```python
from build123d import *

# Parameters (mm, degrees)
BOSS_EXTRUDE1_DEPTH     = 20
BOSS_EXTRUDE2_START     = -5
BOSS_EXTRUDE2_DEPTH     = 5
CUT_EXTRUDE1_DEPTH      = 295.553899991
CUT_EXTRUDE1_DEPTH_BACK = 295.553899991
SKETCH3_R               = 1.5
SKETCH4_R               = 29
BOSS_EXTRUDE3_DEPTH     = 3
SKETCH5_R               = 18.5
CUT_EXTRUDE2_DEPTH      = 4
CUT_EXTRUDE3_DEPTH      = 295.623488541
CUT_EXTRUDE3_DEPTH_BACK = 295.623488541
SKETCH6_R               = 15.5
FILLET1_R               = 10
CUT_EXTRUDE4_DEPTH      = 295.553899998
CUT_EXTRUDE4_DEPTH_BACK = 295.553899998
SKETCH7_R               = 10


with BuildPart() as part:
    # Sketch1 → Boss-Extrude1 (new body)
    with BuildSketch(Plane(origin=(0, 0, 0), x_dir=(1, 0, 0), z_dir=(0, 1, 0))):
        with BuildLine():
            Line((0, -41), (250, -41))
            ThreePointArc((250, -41), (291, 0), (250, 41))
            Line((250, 41), (0, 41))
            ThreePointArc((0, 41), (-41, 0), (0, -41))
        make_face()
        with BuildLine():
            Line((0, 29), (250, 29))
            ThreePointArc((250, 29), (279, 0), (250, -29))
            Line((250, -29), (0, -29))
            ThreePointArc((0, -29), (-29, 0), (0, 29))
        make_face(mode=Mode.SUBTRACT)
    extrude(amount=BOSS_EXTRUDE1_DEPTH)

    # Sketch1<2> → Boss-Extrude2 (add)
    with BuildSketch(Plane(origin=(0, 0, 0), x_dir=(1, 0, 0), z_dir=(0, 1, 0)).offset(BOSS_EXTRUDE2_START)):
        with BuildLine():
            ThreePointArc((0, 41), (-41, 0), (0, -41))
            Line((0, -41), (250, -41))
            ThreePointArc((250, -41), (291, 0), (250, 41))
            Line((250, 41), (0, 41))
        make_face()
    extrude(amount=BOSS_EXTRUDE2_DEPTH)

    # Sketch3 → Cut-Extrude1 (cut, two sides: drawn at the far end of the back side and taken through both)
    with BuildSketch(Plane(origin=(0, 0, 0), x_dir=(1, 0, 0), z_dir=(0, 1, 0)).offset(-CUT_EXTRUDE1_DEPTH_BACK)):
        with Locations(Location((0, 15, 0), (0, 0, 270))):
            Circle(SKETCH3_R)
        with Locations(Location((15, 0, 0), (0, 0, 270))):
            Circle(SKETCH3_R)
        with Locations(Location((0, -15, 0), (0, 0, 270))):
            Circle(SKETCH3_R)
        with Locations(Location((-15, 0, 0), (0, 0, 270))):
            Circle(SKETCH3_R)
    extrude(amount=CUT_EXTRUDE1_DEPTH + CUT_EXTRUDE1_DEPTH_BACK, mode=Mode.SUBTRACT)

    # Sketch4 → Boss-Extrude3 (add)
    with BuildSketch(Plane(origin=(0, 0, 0), x_dir=(1, 0, 0), z_dir=(0, 1, 0))):
        with Locations((250, 0)):
            Circle(SKETCH4_R)
    extrude(amount=BOSS_EXTRUDE3_DEPTH)

    # Sketch5 → Cut-Extrude2 (cut)
    with BuildSketch(Plane(origin=(0, 3, 0), x_dir=(1, 0, 0), z_dir=(0, 1, 0))):
        with Locations(Location((250, 0, 0), (0, 0, 270))):
            Circle(SKETCH5_R)
    extrude(amount=-CUT_EXTRUDE2_DEPTH, mode=Mode.SUBTRACT)

    # Sketch6 → Cut-Extrude3 (cut, two sides: drawn at the far end of the back side and taken through both)
    with BuildSketch(Plane(origin=(0, -1, 0), x_dir=(1, 0, 0), z_dir=(0, 1, 0)).offset(-CUT_EXTRUDE3_DEPTH_BACK)):
        with Locations(Location((250, 0, 0), (0, 0, 270))):
            Circle(SKETCH6_R)
    extrude(amount=CUT_EXTRUDE3_DEPTH + CUT_EXTRUDE3_DEPTH_BACK, mode=Mode.SUBTRACT)

    # Fillet1
    # the kernel refuses this fillet: 10 mm, written as the material it adds along each edge
    with BuildSketch(Plane(origin=(250, 0, 0), x_dir=(0.5782894613752282, 0, -0.8158316608604672), z_dir=(0.8158316608604672, 0, 0.5782894613752282))) as fillet1_piece_1:
        with BuildLine():
            CenterArc((36.141428429, 10), FILLET1_R, 224.427004001, 45.572995999)
            Line((36.141428429, 0), (36.141428429, -0.2))
            Line((36.141428429, -0.2), (29, -0.2))
            Line((29, -0.2), (28.8, 0))
            ThreePointArc((28.8, 0), (28.8, 1.5), (28.857171431, 2.86))
            Line((28.857171431, 2.86), (29, 3))
        make_face()
    revolve(axis=Axis((250, 0, 0), (0, 1, 0)), revolution_arc=250.660644369)

    # Sketch7 → Cut-Extrude4 (cut, two sides: drawn at the far end of the back side and taken through both)
    with BuildSketch(Plane(origin=(0, 0, 0), x_dir=(1, 0, 0), z_dir=(0, 1, 0)).offset(-CUT_EXTRUDE4_DEPTH_BACK)):
        with Locations(Location((70.3, 0, 0), (0, 0, 270))):
            Circle(SKETCH7_R)
    extrude(amount=CUT_EXTRUDE4_DEPTH + CUT_EXTRUDE4_DEPTH_BACK, mode=Mode.SUBTRACT)


solid = part.part
```
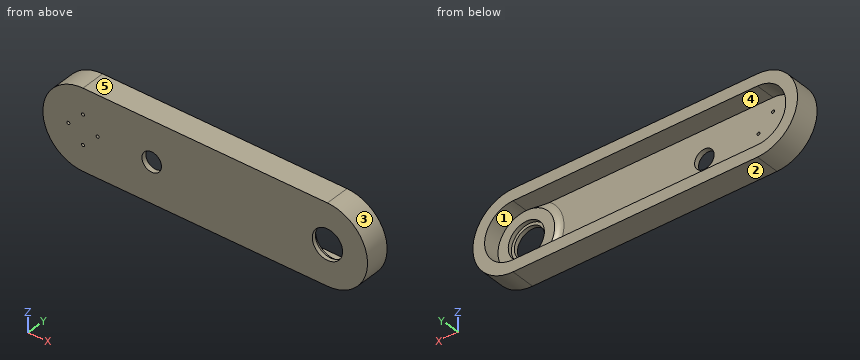
Design review of the part built by this model. Coordinates are the model's own, in mm. Face numbers are marked on the shaded views. A direction names the side the tool comes from. Coordinates: 2 decimals unless noted, no trailing zeros. Loops run counter-clockwise (first coordinate to the right, second up) from the corner with the lowest first, then second, coordinate; pieces in that order, holes last. Notation, with made-up numbers: (49, 0) - (94, 0) arc R32 ccw to (94, 35) - close; hole circle Ø1 at (70.25, 38). An arc over 180 degrees is marked (long way). Use CSV: the item, a comma, the result in double quotes. Start each with the question number.
1) The part is to be moulded in two halves that separate along Z. For the marked faces 3, 4 and 5, say which applies: +Z half, -Z half, draft (parallel to the pull), parting line (faces both ways), or undercut.
2) Wall thickness on L1, parallel to X at y = -2.25, z = 0; L2, parallel to Z at x = 17.5, y = 11.75; L3, parallel to X at y = 2.25, z = -10: over which ranges is each line inside the solid? List them lowest first. Write a range as from..to.
3) Consider section C-C on x = -19.5. Write out the cut boundary in (y, z), then the cut area to 3 significant figures.
4) Consider section A-A on x = 70.3. Write out the cut boundary in (y, z).
5) For pin 1 Ø3.5 at (x, z) = (-15, 0) entering from -Y; pin 2 Ø2.5 at (x, z) = (0, -15) entering from +Y; pin 3 Ø2 at (x, y) = (254.5, 5) entering from -Z; pin 4 Ø1.5 at (x, z) = (170, -4.5) entering from +Y, all flat-tipped, find the tip position at first contact; note any pin that passes through.
6) Consider section B-B on y = 16.5. Write out the cut boundary in (x, z), then the cut area to 3 significant figures.
7) Tool access review of the marked faces 1 and 2: name each direction out of +Z, -Z, +X, -X, +Y, -Y from which nothing blocks a thin tool from reaching the whole face with its end or side.
Geometry says:
1,face 3,"parting line"
1,face 4,"undercut"
1,face 5,"+Z half"
2,L1,"-41..-16.5, -13.5..13.5, 16.5..60.3, 80.3..234.5, 265.5..291"
2,L2,"-41..-29, 29..41"
2,L3,"-39.76..-27.22, 221.9..234.44, 265.56..289.76"
3,outline,"(-5, -36.07) - (20, -36.07) - (20, -21.47) - (0, -21.47) - (0, 21.47) - (20, 21.47) - (20, 36.07) - (-5, 36.07) - close"
3,area,"945 mm^2"
4,outline,"(-5, -41) - (20, -41) - (20, -29) - (0, -29) - (0, -10) - (-5, -10) - close; (-5, 10) - (0, 10) - (0, 29) - (20, 29) - (20, 41) - (-5, 41) - close"
5,pin 1,"y = -5"
5,pin 2,"through"
5,pin 3,"z = -40.85"
5,pin 4,"y = 0"
6,outline,"(0, -41) - (250, -41) arc R41 ccw to (250, 41) - (0, 41) arc R41 ccw to start; hole (0, -29) - (250, -29) arc R29 ccw to (250, 29) - (0, 29) arc R29 ccw to start"
6,area,"8,640 mm^2"
7,face 1,"+Y"
7,face 2,"-Z, +X, -X, +Y, -Y"
